Study the drawing (mm; zero at the part's minimum x, y, z) and answer. Give positions to 0.01 mm unless a question says otherwise; leave off trailing zeros. Order: outer loops, then holes, each group sorted by start corner. A loop starts at its lowest first (then second) coordinate and runs counter-clockwise, first axis right, second up. Notation, with made-up numbers: (-15, -32.75) -> (11, -32.75) arc R21 cw to (11, -11.75) -> close; hole circle Ø1 at (14, -4). An arc over 180 degrees is marked (long way). One line per question, with ' | ' between items. Start each with the question number.
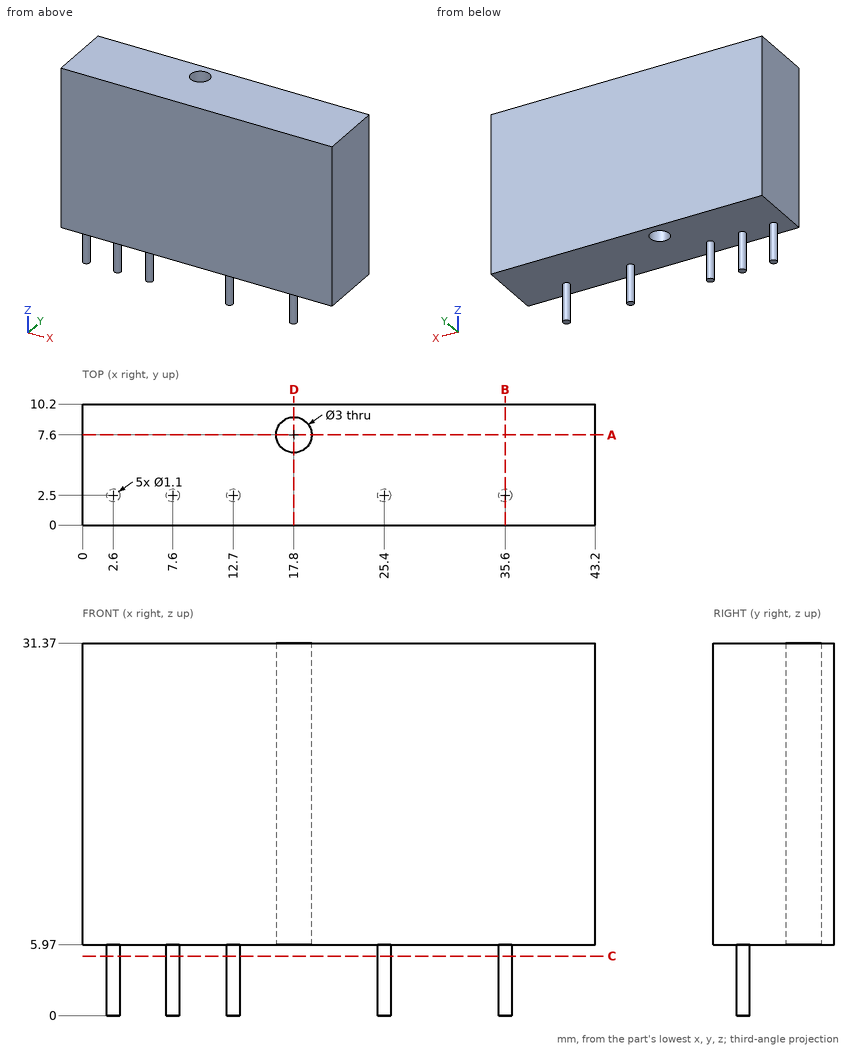
Q1. A cutting plane is placed at B-B, the plane x = 35.6. Determine the outline of the cut face in (y, z), then the cut area to 3 significant figures.
Q2. Given P1, Ø5, axis at x = 18.5, y = 4.5, coming from the -Z side, flat-ended and moving along its own axis, determine where the tip first touches the part or whether it passes through.
Q3. Find the intervals of material crossed by line 1 (Y direction, x = 17.8, z = 18); line 2 (X direction, y = 7.6, z = 23.25); line 3 (Z direction, x = 29.5, y = 3.75), in increasing order.
Q4. A cutting plane is placed at A-A, the plane y = 7.6. Determine the outline of the cut face in (x, z).
Q5. A cutting plane is placed at D-D, the plane x = 17.8. Determine the outline of the cut face in (y, z), then the cut area to 3 significant figures.
Q6. A cutting plane is placed at C-C, the plane z = 5. Determine the outline of the cut face in (x, y).
Geometry results:
1) outline: (0, 5.97) -> (1.95, 5.97) -> (1.95, 0) -> (3.05, 0) -> (3.05, 5.97) -> (10.2, 5.97) -> (10.2, 31.37) -> (0, 31.37) -> close | area: 266 mm²
2) P1: z = 5.97
3) line 1: 0 to 6.1, 9.1 to 10.2 | line 2: 0 to 16.3, 19.3 to 43.2 | line 3: 5.97 to 31.37
4) outline: (0, 5.97) -> (16.3, 5.97) -> (16.3, 31.37) -> (0, 31.37) -> close; (19.3, 5.97) -> (43.2, 5.97) -> (43.2, 31.37) -> (19.3, 31.37) -> close
5) outline: (0, 5.97) -> (6.1, 5.97) -> (6.1, 31.37) -> (0, 31.37) -> close; (9.1, 5.97) -> (10.2, 5.97) -> (10.2, 31.37) -> (9.1, 31.37) -> close | area: 183 mm²
6) outline: circle Ø1.1 at (2.6, 2.5); circle Ø1.1 at (7.6, 2.5); circle Ø1.1 at (12.7, 2.5); circle Ø1.1 at (25.4, 2.5); circle Ø1.1 at (35.6, 2.5)
